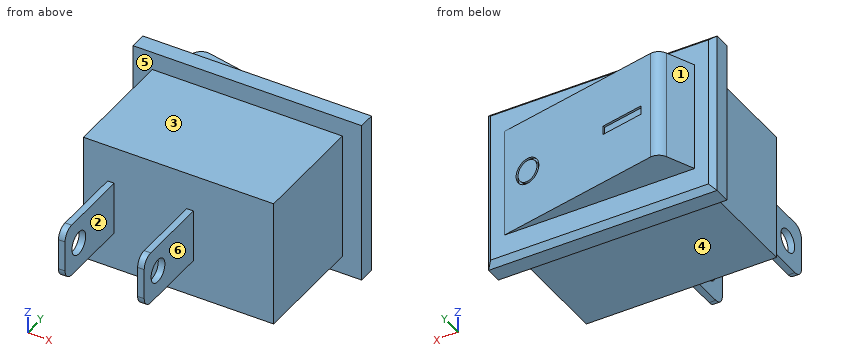
```python
from build123d import *

# Parameters (mm, degrees)
SKETCH_1_W          = 17.3
SKETCH_1_H          = 11.6
EXTRUDE_1_DEPTH     = 10.5
SKETCH_2_W          = 20.8
SKETCH_2_H          = 14.9
EXTRUDE_2_DEPTH     = 2
CHAMFER_1_SIZE      = 0.5
SKETCH_3_W          = 0.6
SKETCH_3_H          = 4.8
EXTRUDE_3_DEPTH     = 7.5
SKETCH_4_R          = 1.05
CUT_EXTRUDE_1_DEPTH = 17.85
FILLET_1_R          = 1
EXTRUDE_4_DEPTH     = 5
SKETCH_7_R          = 1.2
SKETCH_7_R_2        = 1
SKETCH_7_W          = 4
SKETCH_7_H          = 0.8
CUT_EXTRUDE_2_DEPTH = 0.2


with BuildPart() as part:
    # 草图1 → 凸台-拉伸1 (new body)
    with BuildSketch(Plane(origin=(0, 0, 0), x_dir=(1, 0, 0), z_dir=(0, 1, 0))):
        Rectangle(SKETCH_1_W, SKETCH_1_H)
    extrude(amount=EXTRUDE_1_DEPTH)

    # 草图2 → 凸台-拉伸2 (add)
    with BuildSketch(Plane(origin=(0, 10.5, 0), x_dir=(1, 0, 0), z_dir=(0, 1, 0))):
        Rectangle(SKETCH_2_W, SKETCH_2_H)
    extrude(amount=EXTRUDE_2_DEPTH)

    # 倒角1
    chamfer_1_edges = [part.edges().sort_by_distance(p)[0] for p in [
        (10.4, 12.5, 0),
        (0, 12.5, -7.45),
        (-10.4, 12.5, 0),
        (0, 12.5, 7.45),
    ]]
    chamfer(chamfer_1_edges, length=CHAMFER_1_SIZE)

    # 草图3 → 凸台-拉伸3 (add)
    with BuildSketch(Plane.XZ):
        with Locations((-6.15, 0)):
            Rectangle(SKETCH_3_W, SKETCH_3_H)
        with Locations((1.05, 0)):
            Rectangle(SKETCH_3_W, SKETCH_3_H)
    extrude(amount=EXTRUDE_3_DEPTH)

    # 草图4 → 切除-拉伸1 (cut, through all)
    with BuildSketch(Plane.ZY.offset(6.45)):
        with Locations((0, -5.4)):
            Circle(SKETCH_4_R)
    extrude(amount=-CUT_EXTRUDE_1_DEPTH, mode=Mode.SUBTRACT)

    # 圆角1
    fillet_1_edges = [part.edges().sort_by_distance(p)[0] for p in [
        (-6.15, -7.5, -2.4),
        (-6.15, -7.5, 2.4),
        (1.05, -7.5, -2.4),
        (1.05, -7.5, 2.4),
    ]]
    fillet(fillet_1_edges, radius=FILLET_1_R)

    # 草图6 → 凸台-拉伸4 (add, symmetric)
    with BuildSketch(Plane.XY):
        with BuildLine():
            Line((-8.65, 12.5), (-7.567226169, 14.993049988))
            ThreePointArc((-7.567226169, 14.993049988), (-7.111867175, 15.481632233), (-6.450485665, 15.574578036))
            Line((-6.450485665, 15.574578036), (8.65, 12.5))
            Line((8.65, 12.5), (9.9, 12.5))
            Line((9.9, 12.5), (10.4, 12))
            Line((10.4, 12), (-10.4, 12))
            Line((-10.4, 12), (-9.9, 12.5))
            Line((-9.9, 12.5), (-8.65, 12.5))
        make_face()
    extrude(amount=EXTRUDE_4_DEPTH, both=True)

    # 草图7 → 切除-拉伸2 (cut)
    with BuildSketch(Plane(origin=(2.788110156, 13.693527027, 0), x_dir=(0.979894908, -0.199514335, 0), z_dir=(0.199514335, 0.979894908, 0))):
        with Locations((3.54609821, 0)):
            Circle(SKETCH_7_R)
        with Locations((3.54609821, 0)):
            Circle(SKETCH_7_R_2, mode=Mode.SUBTRACT)
        with Locations((-6.42814964, -0.024521247)):
            Rectangle(SKETCH_7_W, SKETCH_7_H)
    extrude(amount=-CUT_EXTRUDE_2_DEPTH, mode=Mode.SUBTRACT)


solid = part.part
```
Check sheet for the modelled part. Datum: model origin and axes. Units: mm. Face numbers are marked on the shaded views. A direction names the side the tool comes from. Give positions to 0.01 mm unless a question says otherwise; leave off trailing zeros. Order: outer loops, then holes, each group sorted by start corner. A loop starts at its lowest first (then second) coordinate and runs counter-clockwise, first axis right, second up. Notation, with made-up numbers: M 60.5,28 L 115.5,28 A20 ccw 115.5,57 Z; hole C 76.5,73 d6. An arc over 180 degrees is marked long. Answer in a Markdown table with one row per item. Add a question column.
Q1. Gauge pin test, flat ends, axial feed: pin 1 Ø8 at (x, z) = (-0.5, -1.5) entering from -Y; pin 2 Ø5 at (y, z) = (6.5, 0) entering from -X; pin 3 Ø3 at (x, z) = (0.5, -4) entering from -Y; pin 4 Ø1.9 at (y, z) = (-5.4, 0) entering from -X. Record the tip position at first contact, or that the pin passes through.
Q2. Thickness scan on L1, parallel to Z at x = -4.5, y = 14.75; L2, parallel to Y at x = -9, z = -2; L3, parallel to X at y = 3.25, z = 1.5. Record the ranges inside material, lowest first.
Q3. Release check for a two-part mould opening along X. For the marked faces 1, 2 and 3 record: released by +X, released by -X, zero draft, split by the parting line, or undercut.
Q4. Access from +Z, -Z, +X, -X, +Y, -Y to the whole of each face (thin tool, end or side, straight path). Record for the marked faces 4, 5 and 6.
Q5. Sectioned sample at D-D, the plane x = -1. Record the boundary of the cut face in (y, z), and give its area (3 significant figures).
Q6. Sectioned sample at C-C, the plane y = -5.4. Record the boundary of the cut face in (x, z).
Q7. Sectioned sample at B-B, the plane z = 5.5. Record the boundary of the cut face in (x, y).
Q8. Sectioned sample at A-A, the plane y = -0.5. Record the boundary of the cut face in (x, z).
Verdict:
| question | item | result |
|---|---|---|
| 1 | pin 1 | y = -7.5 |
| 1 | pin 2 | x = -8.65 |
| 1 | pin 3 | y = 0 |
| 1 | pin 4 | through |
| 2 | L1 | -5 to 5 |
| 2 | L2 | 10.5 to 12.5 |
| 2 | L3 | -8.65 to 8.65 |
| 3 | face 1 | released by -X |
| 3 | face 2 | undercut |
| 3 | face 3 | zero draft |
| 4 | face 4 | -Z, +X, -X, -Y |
| 4 | face 5 | -Y |
| 4 | face 6 | +Z, -Z, +X, -Y |
| 5 | outline | M 0,-5.8 L 10.5,-5.8 L 10.5,-7.45 L 12,-7.45 L 12.5,-6.95 L 12.5,-5 L 14.46,-5 L 14.46,5 L 12.5,5 L 12.5,6.95 L 12,7.45 L 10.5,7.45 L 10.5,5.8 L 0,5.8 Z |
| 5 | area | 171 mm² |
| 6 | outline | M -6.45,-2.4 L -5.85,-2.4 L -5.85,-1.05 L -6.45,-1.05 Z; M -6.45,1.05 L -5.85,1.05 L -5.85,2.4 L -6.45,2.4 Z; M 0.75,-2.4 L 1.35,-2.4 L 1.35,-1.05 L 0.75,-1.05 Z; M 0.75,1.05 L 1.35,1.05 L 1.35,2.4 L 0.75,2.4 Z |
| 7 | outline | M -10.4,10.5 L -8.65,10.5 L -8.65,0 L 8.65,0 L 8.65,10.5 L 10.4,10.5 L 10.4,12 L 9.9,12.5 L -9.9,12.5 L -10.4,12 Z |
| 8 | outline | M -6.45,-2.4 L -5.85,-2.4 L -5.85,2.4 L -6.45,2.4 Z; M 0.75,-2.4 L 1.35,-2.4 L 1.35,2.4 L 0.75,2.4 Z |
